CAD build for the part. Positions are in the model's coordinates, mm. Face numbers are marked on the shaded views. A direction names the side the tool comes from. Round coordinates to 2 decimals unless told otherwise and drop trailing zeros. Loops run counter-clockwise (first coordinate to the right, second up) from the corner with the lowest first, then second, coordinate; pieces in that order, holes last. Notation, with made-up numbers: (58, 39.25) -> (69, 39.25) arc R11 ccw to (69, 50.25) -> close; hole circle Ø4 at (39.5, -34.5). An arc over 180 degrees is marked (long way). Answer as CSV lines item,"result".
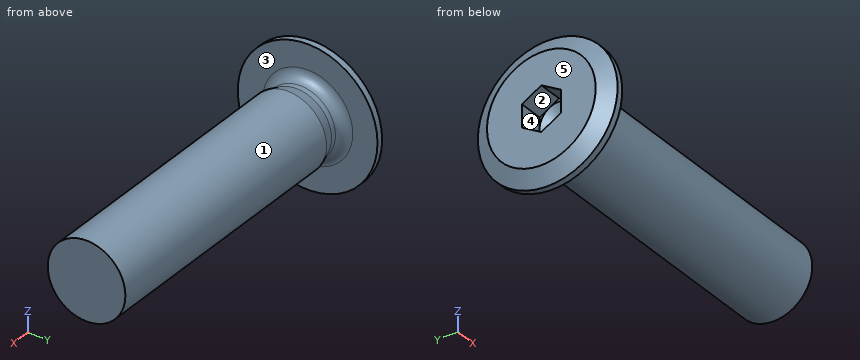
```python
from build123d import *

# Parameters (mm, degrees)
CUT_EXTRUDE1_DEPTH = 1.6
FILLET1_R          = 0.65


with BuildPart() as part:
    # Sketch1 → Revolve1 (revolve)
    with BuildSketch(Plane.XY):
        Polygon((-1, 0), (20, 0), (20, 2.5), (1.8, 2.5), (1, 2.255), (0, 2.255), (0, 4.5), (-0.422649731, 4.5), (-1, 3.5), align=None)
    revolve(axis=Axis((-1, 0, 0), (1, 0, 0)))

    # Sketch2 → Cut-Extrude1 (cut)
    with BuildSketch(Plane.ZY.offset(1)):
        Polygon((-1.443375673, 0), (-0.721687836, -1.25), (0.721687836, -1.25), (1.443375673, 0), (0.721687836, 1.25), (-0.721687836, 1.25), align=None)
    extrude(amount=-CUT_EXTRUDE1_DEPTH, mode=Mode.SUBTRACT)

    # Sketch3 → Cut-Revolve1 (revolve, cut)
    with BuildSketch(Plane.XY):
        Polygon((0.6, -1.25), (0.6, 0), (1.351075774, 0), align=None)
    revolve(axis=Axis((0, 0, 0), (-1, 0, 0)), mode=Mode.SUBTRACT)

    # Fillet1
    fillet1_edges = [part.edges().sort_by_distance(p)[0] for p in [
        (0, -2.255, 0),
    ]]
    fillet(fillet1_edges, radius=FILLET1_R)


solid = part.part
```
Q1. Probe L1, parallel to X at y = 2.75, z = 0.75; L2, parallel to Z at x = 11.5, y = 0; L3, parallel to Y at x = 7.5, z = -2.25. List the from-to ranges inside material, lowest first. Write a range as [from, to].
Results:
L1,"[-1, 0]"
L2,"[-2.5, 2.5]"
L3,"[-1.09, 1.09]"
Q2. Two-plate mould, pull along Z, no slides. Class the marked faces 1, 2 and 3: pulls with the +Z half, pulls with the -Z half, needs draft (parallel to the pull), parting line crosses it, or undercut.
Results:
face 1,"parting line crosses it"
face 2,"undercut"
face 3,"needs draft"
Q3. Drop flat-ended pins along their axis: pin 1 Ø1.5 at (x, y) = (14, -1) entering from +Z; pin 2 Ø1.5 at (x, z) = (4.5, 2.5) entering from +Y; pin 3 Ø5 at (x, z) = (11.5, 1.5) entering from +Y; pin 4 Ø0.7 at (y, z) = (1, 0.5) entering from -X. Give the stop position or say it passes through.
Results:
pin 1,"z = 2.49"
pin 2,"y = 1.79"
pin 3,"y = 2.5"
pin 4,"x = -1"
Q4. Slice it at A-A, the plane x = 16. Give the cut face in (y, z).
Results:
outline,"circle Ø5 at (0, 0)"
Q5. Tool access for the marked faces 4 and 5: list every direction of +Z, -Z, +X, -X, +Y, -Y with a clear straight run to the whole face (end or side of a thin tool).
Results:
face 4,"-X"
face 5,"+Z, -Z, -X, +Y, -Y"
